```python
from build123d import *

# Parameters (mm, degrees)
SKETCH1_R            = 40
BOSS_EXTRUDE11_DEPTH = 5
SKETCH1_14_R         = 1.5
CUT_EXTRUDE5_DEPTH   = 57.789083458
OFFSETCIRCLE_R       = 22.5
BOSS_EXTRUDE14_DEPTH = 10
SKETCH1_15_R         = 22.5
SKETCH1_15_R_2       = 19.5
CUT_EXTRUDE6_DEPTH   = 2.3
SKETCH1_16_R         = 29
SKETCH1_16_R_2       = 25.5
CUT_EXTRUDE7_DEPTH   = 2.5
SKETCH10_R           = 1
CUT_EXTRUDE8_DEPTH   = 58.445626465
SKETCH1_17_R         = 16
CUT_EXTRUDE9_DEPTH   = 5
FILLET1_R            = 0.5
FILLET2_R            = 0.5
FILLET3_R            = 0.5


with BuildPart() as part:
    # Sketch1 → Boss-Extrude11 (new body)
    with BuildSketch(Plane(origin=(0, 0, 0), x_dir=(1, 0, 0), z_dir=(0, 1, 0))):
        with Locations(Location((0, 0, 0), (0, 0, 270))):
            Circle(SKETCH1_R)
    extrude(amount=-BOSS_EXTRUDE11_DEPTH)

    # Sketch1_14 → Cut-Extrude5 (cut, through all)
    with BuildSketch(Plane(origin=(0, 0, 0), x_dir=(1, 0, 0), z_dir=(0, 1, 0))):
        with Locations(Location((35.5, 0, 0), (0, 0, 270))):
            Circle(SKETCH1_14_R)
        with Locations(Location((0, -35.5, 0), (0, 0, 270))):
            Circle(SKETCH1_14_R)
        with Locations(Location((-35.5, 0, 0), (0, 0, 270))):
            Circle(SKETCH1_14_R)
        with Locations(Location((0, 35.5, 0), (0, 0, 270))):
            Circle(SKETCH1_14_R)
    extrude(amount=-CUT_EXTRUDE5_DEPTH, mode=Mode.SUBTRACT)

    # offsetCircle → Boss-Extrude14 (add)
    with BuildSketch(Plane(origin=(0, 0, 0), x_dir=(1, 0, 0), z_dir=(0, 1, 0))):
        with Locations(Location((0, 0, 0), (0, 0, 270))):
            Circle(OFFSETCIRCLE_R)
    extrude(amount=-BOSS_EXTRUDE14_DEPTH)

    # Sketch1_15 → Cut-Extrude6 (cut)
    with BuildSketch(Plane(origin=(0, 0, 0), x_dir=(1, 0, 0), z_dir=(0, 1, 0))):
        with Locations(Location((0, 0, 0), (0, 0, 270))):
            Circle(SKETCH1_15_R)
        with Locations(Location((0, 0, 0), (0, 0, 270))):
            Circle(SKETCH1_15_R_2, mode=Mode.SUBTRACT)
    extrude(amount=-CUT_EXTRUDE6_DEPTH, mode=Mode.SUBTRACT)

    # Sketch1_16 → Cut-Extrude7 (cut)
    with BuildSketch(Plane(origin=(0, 0, 0), x_dir=(1, 0, 0), z_dir=(0, 1, 0))):
        with Locations(Location((0, 0, 0), (0, 0, 270))):
            Circle(SKETCH1_16_R)
        with Locations(Location((0, 0, 0), (0, 0, 270))):
            Circle(SKETCH1_16_R_2, mode=Mode.SUBTRACT)
    extrude(amount=-CUT_EXTRUDE7_DEPTH, mode=Mode.SUBTRACT)

    # Sketch10 → Cut-Extrude8 (cut, through all)
    with BuildSketch(Plane(origin=(0, 0, 0), x_dir=(1, 0, 0), z_dir=(0, 1, 0))):
        with Locations(Location((29, 22.5, 0), (0, 0, 270))):
            Circle(SKETCH10_R)
    extrude(amount=-CUT_EXTRUDE8_DEPTH, mode=Mode.SUBTRACT)

    # Sketch1_17 → Cut-Extrude9 (cut)
    with BuildSketch(Plane(origin=(0, 0, 0), x_dir=(1, 0, 0), z_dir=(0, 1, 0))):
        with Locations(Location((0, 0, 0), (0, 0, 270))):
            Circle(SKETCH1_17_R)
    extrude(amount=-CUT_EXTRUDE9_DEPTH, mode=Mode.SUBTRACT)

    # Fillet1
    fillet1_edges = [part.edges().sort_by_distance(p)[0] for p in [
        (0, -5, -40),
    ]]
    fillet(fillet1_edges, radius=FILLET1_R)

    # Fillet2
    fillet2_edges = [part.edges().sort_by_distance(p)[0] for p in [
        (0, 0, -40),
    ]]
    fillet(fillet2_edges, radius=FILLET2_R)

    # Fillet3
    fillet3_edges = [part.edges().sort_by_distance(p)[0] for p in [
        (0, -10, -22.5),
    ]]
    fillet(fillet3_edges, radius=FILLET3_R)


solid = part.part
```
CAD build for the part. Positions are in the model's coordinates, mm. A direction names the side the tool comes from. Round coordinates to 2 decimals unless told otherwise and drop trailing zeros. Order: outer loops, then holes, each group sorted by start corner. A loop starts at its lowest first (then second) coordinate and runs counter-clockwise, first axis right, second up.
Item 1: Tool access for faces 4 (the face through (-17, -5, 17)), 5 (the face through (34, -2, 0)), 6 (the face through (19.334, -1.134, -2.539)): list every direction of +Z, -Z, +X, -X, +Y, -Y with a clear straight run to the whole face (end or side of a thin tool).
Item 2: Pin check, flat tips, straight feed: pin 1 (1.8 mm diameter, centred on x = -35.5, z = 0, fed in from +Y); pin 2 (16 mm diameter, centred on x = 6.5, z = -0.5, fed in from +Y); pin 3 (5 mm diameter, centred on x = 14, z = -19.5, fed in from +Y); pin 4 (6 mm diameter, centred on x = 15, y = -1, fed in from -Z). Stop position of each tip, or through.
Item 3: Saw through at A-A on y = -3.5. Write the cut outline in (x, z).
Item 4: Mould opens along X. For faces 1 (the face through (-26, -2.5, 0)), 2 (the face through (-39.05, -2.47, -8.67)), 3 (the face through (0, -10, 0)) say: pulls with the +X half, pulls with the -X half, needs draft (parallel to the pull), parting line crosses it, or undercut.
Item 5: Probe line 1 along X through (y, z) = (-1.5, 9); line 2 along X through (y, z) = (-1, 7); line 3 along Y through (x, z) = (28, 21). List the from-to ranges inside material, lowest first.
Item 6: Saw through at B-B on x = 0. State how many separate pieces and enclosed holes the cut face has, then the cut area to 3 significant figures.
Reported:
1. face 4: -Y
1. face 5: +Y, -Y
1. face 6: +Y
2. pin 1: passes through
2. pin 2: stops at y = -5
2. pin 3: stops at y = 0
2. pin 4: stops at z = -38.16
3. outline: circle Ø80 at (0, 0); hole circle Ø3 at (-35.5, 0); hole circle Ø32 at (0, 0); hole circle Ø3 at (0, -35.5); hole circle Ø3 at (0, 35.5); hole circle Ø2 at (29, -22.5); hole circle Ø3 at (35.5, 0)
4. face 1: undercut
4. face 2: parting line crosses it
4. face 3: needs draft
5. line 1: x = -38.97 to -27.57, -23.86 to -20.62, -17.3 to -13.23, 13.23 to 17.3, 20.62 to 23.86, 27.57 to 38.97
5. line 2: x = -39.38 to -28.14, -24.52 to -21.38, -18.2 to -14.39, 14.39 to 18.2, 21.38 to 24.52, 28.14 to 39.38
5. line 3: y = -5 to 0
6. separate pieces: 3
6. enclosed holes: 0
6. area: 403 mm2
